Source: CAD feature listing. Evaluate the final solid. Frame: model axes, mm. A direction names the side the tool comes from. Give positions to 0.01 mm unless a question says otherwise; leave off trailing zeros. Loops run counter-clockwise (first coordinate to the right, second up) from the corner with the lowest first, then second, coordinate; pieces in that order, holes last. Notation, with made-up numbers: M 9.25,53 L 43.25,53 A30 cw 43.25,88 Z; hole C 4,8 d5. An arc over 180 degrees is marked long. Answer in a Markdown table with one row per item.
Autodesk Inventor part; units mm, degrees
ref_plane "YZ Plane" through (0, 0, 0) normal (1, 0, 0) x (0, 1, 0)
ref_plane "XZ Plane" through (0, 0, 0) normal (0, 1, 0) x (-1, 0, 0)
ref_plane "XY Plane" through (0, 0, 0) normal (0, 0, 1) x (1, 0, 0)
sketch "Sketch1" plane through (0, 0, 0) normal (0, 0, 1) x (1, 0, 0)
  line L0 (0, 0) -> (0, 90)
  line L1 (0, 90) -> (19.2, 90)
  line L2 (19.2, 90) -> (19.2, 56)
  line L3 (19.2, 56) -> (35.07, 56)
  line L4 (35.07, 56) -> (35.07, 90)
  line L5 (35.07, 90) -> (54.27, 90)
  line L6 (54.27, 90) -> (54.27, 0)
  line L7 (54.27, 0) -> (35.07, 0)
  line L8 (35.07, 0) -> (35.07, 34)
  line L9 (35.07, 34) -> (19.2, 34)
  line L10 (19.2, 34) -> (19.2, 0)
  line L11 (0, 0) -> (19.2, 0)
  dimension "d0" = 90
  dimension "d1" = 19.2
  dimension "d2" = 34
  dimension "d3" = 15.87
  dimension "d4" = 19.2
  dimension "d5" = 34
  dimension "d37" = 22
extrude "Extrusion1" add sketch "Sketch1" along normal blind 20.67
sketch "Sketch2" plane through (19.2, 56, 0) normal (0, 1, 0) x (1, 0, 0)
  line L0 (15.87, 0) -> (0, 0)
  line L1 (11.39, 0) -> (4.49, 0)
  line L2 (4.49, 0) -> (4.49, -4.29)
  line L3 (4.49, -4.29) -> (11.39, -4.29)
  line L4 (11.39, -4.29) -> (11.39, 0)
  point P0 (-19.2, 0)
  dimension "d8" = 6.9
  dimension "d9" = 4.29
extrude "Extrusion2" add sketch "Sketch2" along normal blind 27.15
sketch "Sketch3" plane through (23.69, 56, 4.29) normal (0, 0, 1) x (1, 0, 0)
  line L0 (6.9, 0) -> (0, 0)
  line L1 (0, 27.15) -> (6.9, 27.15)
  line L2 (0, 0) -> (0, 27.15)
  line L3 (6.9, 27.15) -> (9.7769, 2.4369)
  line L4 (6.9, 27.15) -> (31.78, 27.15) construction
  line L5 (9.7769, 2.4369) -> (6.9, 2.4369)
  line L6 (6.9, 0) -> (6.9, 27.15)
  line L7 (0, 2.4369) -> (-2.877, 2.4369)
  line L8 (-2.877, 2.4369) -> (0, 27.15)
  point P0 (-23.69, -56)
  dimension "d12" = 24.88
  dimension "d13" = 83.36
  dimension "d14" = 2.877
extrude "Extrusion3" add sketch "Sketch3" against normal blind 4.29
sketch "Sketch4" plane through (19.2, 34, 0) normal (0, -1, 0) x (1, 0, 0)
  line L0 (0, 0) -> (0, 20.67)
  line L1 (0, 0) -> (4.49, 0)
  line L2 (4.48, 0) -> (11.38, 0)
  line L3 (11.38, 0) -> (11.38, 4.29)
  line L4 (11.38, 4.29) -> (4.48, 4.29)
  line L5 (4.48, 4.29) -> (4.48, 0)
  point P0 (-19.2, 0)
  dimension "d17" = 6.9
  dimension "d18" = 4.29
  dimension "d19" = 4.48
extrude "Extrusion4" add sketch "Sketch4" along normal blind 18.76
sketch "Sketch5" plane through (23.68, 34, 4.29) normal (0, 0, 1) x (1, 0, 0)
  line L0 (0, 0) -> (6.9, 0)
  line L1 (0, 0) -> (0, -18.76)
  line L2 (6.9, -18.76) -> (0, -18.76)
  line L3 (0, -18.76) -> (-2.87, -2.3288)
  line L4 (-4.48, -34) -> (-4.48, 0)
  line L5 (-2.87, -2.3288) -> (0, -2.3288)
  line L6 (6.9, 0) -> (6.9, -18.76)
  line L7 (6.9, -2.3288) -> (9.777, -2.3288)
  line L8 (9.777, -2.3288) -> (6.9, -18.76)
  point P0 (-23.68, -34)
  dimension "d22" = 16.68
  dimension "d23" = 1.61
  dimension "d24" = 2.877
extrude "Extrusion5" add sketch "Sketch5" against normal blind 4.29
sketch "Sketch6" plane through (0, 0, 20.67) normal (0, 0, 1) x (1, 0, 0)
  line L0 (0.93, 0.93) -> (0.93, 89.07)
  line L1 (0, 90) -> (19.2, 90)
  line L2 (0.93, 89.07) -> (18.27, 89.07)
  line L3 (18.27, 89.07) -> (18.27, 55.07)
  line L4 (18.27, 55.07) -> (36, 55.07)
  line L5 (36, 55.07) -> (36, 89.07)
  line L6 (36, 89.07) -> (53.34, 89.07)
  line L7 (53.34, 89.07) -> (53.34, 0.93)
  line L8 (53.34, 0.93) -> (36, 0.93)
  line L9 (36, 0.93) -> (36, 34.93)
  line L10 (36, 34.93) -> (18.27, 34.93)
  line L11 (18.27, 34.93) -> (18.27, 0.93)
  line L12 (18.27, 0.93) -> (0.93, 0.93)
  line L13 (35.07, 56) -> (19.2, 56)
  dimension "d27" = 88.14
  dimension "d28" = 17.34
  dimension "d29" = 34
  dimension "d30" = 17.73
  dimension "d31" = 34
  dimension "d32" = 17.34
  dimension "d33" = 88.14
  dimension "d34" = 34
  dimension "d38" = 0.93
  dimension "d39" = 0.93
extrude "Extrusion6" cut sketch "Sketch6" against normal blind 0.62
sketch "Sketch7" plane through (0, 0, 20.05) normal (0, 0, 1) x (1, 0, 0)
  line L0 (0.93, 0.93) -> (0.93, 89.07)
  line L1 (36, 34.93) -> (18.27, 34.93)
  line L2 (53.34, 89.07) -> (53.34, 0.93)
  line L3 (18.27, 55.07) -> (36, 55.07)
  line L4 (17.08, 52.05) -> (37.18, 52.05)
  line L5 (37.18, 52.05) -> (37.18, 37.95)
  line L6 (37.18, 37.95) -> (17.08, 37.95)
  line L7 (17.08, 37.95) -> (17.08, 52.05)
  point P0 (0, 0)
  dimension "d40" = 14.1
  dimension "d41" = 20.1
  dimension "d42" = 3.02
  dimension "d43" = 3.02
  dimension "d44" = 16.15
  dimension "d45" = 16.16
extrude "Extrusion7" cut sketch "Sketch7" against normal blind 12
sketch "Sketch8" plane through (0, 0, 8.05) normal (0, 0, 1) x (1, 0, 0)
  line L0 (17.08, 52.05) -> (37.18, 52.05)
  line L1 (17.08, 37.95) -> (17.08, 52.05)
  line L2 (21.58, 46.35) -> (32.58, 46.35)
  line L3 (32.58, 46.35) -> (32.58, 43.75)
  line L4 (32.58, 43.75) -> (21.58, 43.75)
  line L5 (21.58, 43.75) -> (21.58, 46.35)
  point P0 (0, 0)
  dimension "d48" = 11
  dimension "d49" = 2.6
  dimension "d50" = 5.7
  dimension "d51" = 4.5
extrude "Extrusion8" cut sketch "Sketch8" against normal up to next
properties part number "Gebouw Helix V1"
1) Set-up query: faces 5 (the flat face through (19.2, 17, 10)), 6 (the flat face through (17.08, 45, 14)), 7 (the flat face through (27, 46.35, 4)), 8 (the flat face through (27, 69, 4.29)). Return all of +Z, -Z, +X, -X, +Y, -Y with unobstructed straight access to the full face (end or side cutting, diameter ignored); none if empty.
Reply:
| item | result |
|---|---|
| face 5 | +Z, -Z, -Y |
| face 6 | +Z |
| face 7 | +Z, -Z |
| face 8 | +Z, +Y |
2) Pin query (flat end, axial travel): pin 1 Ø10 at (x, y) = (27, 22.5) entering from +Z; pin 2 Ø4.5 at (x, z) = (26.5, 3) entering from +Y. Return the tip coordinate at first contact, or that it passes through.
Reply:
| item | result |
|---|---|
| pin 1 | stops at z = 4.29 |
| pin 2 | stops at y = 83.15 |
3) Section B-B, the plane z = 10. Return loops of the section in (x, y).
Reply:
| item | result |
|---|---|
| outline | M 0,0 L 19.2,0 L 19.2,34 L 35.07,34 L 35.07,0 L 54.27,0 L 54.27,90 L 35.07,90 L 35.07,56 L 19.2,56 L 19.2,90 L 0,90 Z; hole M 17.08,37.95 L 37.18,37.95 L 37.18,52.05 L 17.08,52.05 Z |
4) Section D-D, the plane y = 54. Return loops of the section in (x, z).
Reply:
| item | result |
|---|---|
| outline | M 0,0 L 54.27,0 L 54.27,20.67 L 53.34,20.67 L 53.34,20.05 L 0.93,20.05 L 0.93,20.67 L 0,20.67 Z |
5) Pull-direction query (X, two-part tool) for faces 1 (the flat face through (9, 90, 10)), 2 (the flat face through (54.27, 46, 10)), 3 (the flat face through (0, 44, 10)), 4 (the flat face through (27, 15.24, 2)); classes: released by +X, released by -X, zero draft, split by the parting line, or undercut.
Reply:
| item | result |
|---|---|
| face 1 | zero draft |
| face 2 | released by +X |
| face 3 | released by -X |
| face 4 | undercut |
6) Section C-C, the plane x = 5.5. Return loops of the section in (y, z), then the cut area to 3 significant figures.
Reply:
| item | result |
|---|---|
| outline | M 0,0 L 90,0 L 90,20.67 L 89.07,20.67 L 89.07,20.05 L 0.93,20.05 L 0.93,20.67 L 0,20.67 Z |
| area | 1,810 mm² |
7) Material intervals for L1, parallel to X at y = 33, z = 16.25; L2, parallel to Y at x = 26, z = 19.25; L3, parallel to X at y = 79, z = 3.75, sorted ascending.
Reply:
| item | result |
|---|---|
| L1 | x = 0 to 19.2, 35.07 to 54.27 |
| L2 | y = 34 to 37.95, 52.05 to 56 |
| L3 | x = 0 to 19.2, 23.21 to 31.07, 35.07 to 54.27 |
8) Section A-A, the plane y = 12.5. Return loops of the section in (x, z).
Reply:
| item | result |
|---|---|
| outline | M 0,0 L 19.2,0 L 19.2,20.67 L 18.27,20.67 L 18.27,20.05 L 0.93,20.05 L 0.93,20.67 L 0,20.67 Z; M 35.07,0 L 54.27,0 L 54.27,20.67 L 53.34,20.67 L 53.34,20.05 L 36,20.05 L 36,20.67 L 35.07,20.67 Z |
